Could you check a few things on this model? Use its own coordinates, in mm. Face numbers are marked on the shaded views. Coordinates: 2 decimals unless noted, no trailing zeros. Order: outer loops, then holes, each group sorted by start corner. A loop starts at its lowest first (then second) coordinate and runs counter-clockwise, first axis right, second up. Notation, with made-up numbers: (24, 50.25) - (54, 50.25) arc R25 ccw to (54, 69.25) - close; hole circle Ø2 at (47.5, 21). An arc over 180 degrees is marked (long way). One line per item, written item: value.
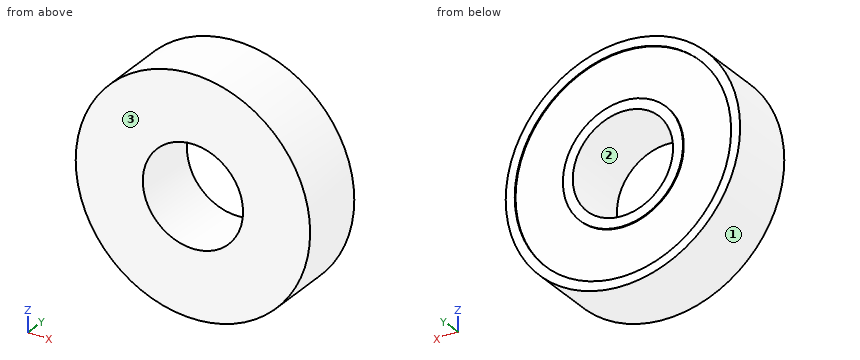
from build123d import *

# Parameters (mm, degrees)
CROQUIS1_R              = 13.975
SALIENTE_EXTRUIR1_DEPTH = 8
CROQUIS2_R              = 5.98
CORTAR_EXTRUIR1_DEPTH   = 8
CROQUIS3_R              = 7.163309877
CROQUIS3_R_2            = 5.98
SALIENTE_EXTRUIR3_DEPTH = 0.15
CROQUIS4_R              = 13.975
CROQUIS4_R_2            = 12.899809837
SALIENTE_EXTRUIR4_DEPTH = 8.15


with BuildPart() as part:
    # Croquis1 → Saliente-Extruir1 (new body)
    with BuildSketch(Plane(origin=(0, 0, 0), x_dir=(1, 0, 0), z_dir=(0, 1, 0))):
        Circle(CROQUIS1_R)
    extrude(amount=SALIENTE_EXTRUIR1_DEPTH)

    # Croquis2 → Cortar-Extruir1 (cut)
    with BuildSketch(Plane(origin=(0, 8, 0), x_dir=(1, 0, 0), z_dir=(0, 1, 0))):
        Circle(CROQUIS2_R)
    extrude(amount=-CORTAR_EXTRUIR1_DEPTH, mode=Mode.SUBTRACT)

    # Croquis3 → Saliente-Extruir3 (add)
    with BuildSketch(Plane(origin=(0, 8, 0), x_dir=(1, 0, 0), z_dir=(0, 1, 0))):
        Circle(CROQUIS3_R)
        Circle(CROQUIS3_R_2, mode=Mode.SUBTRACT)
    extrude(amount=SALIENTE_EXTRUIR3_DEPTH)

    # Croquis4 → Saliente-Extruir4 (add)
    with BuildSketch(Plane(origin=(0, 0, 0), x_dir=(1, 0, 0), z_dir=(0, 1, 0))):
        Circle(CROQUIS4_R)
        Circle(CROQUIS4_R_2, mode=Mode.SUBTRACT)
    extrude(amount=SALIENTE_EXTRUIR4_DEPTH)


solid = part.part
Item 1: I want a section at D-D on z = 8. Please give me the cut outline in (x, y).
Conclusion:
outline: (-11.46, 0) - (11.46, 0) - (11.46, 8.15) - (10.12, 8.15) - (10.12, 8) - (-10.12, 8) - (-10.12, 8.15) - (-11.46, 8.15) - close
Item 2: I want a section at C-C on y = 7. Please give me the cut outline in (x, z) (3 decimals).
Conclusion:
outline: circle Ø27.95 at (0, 0); hole circle Ø11.96 at (0, 0)
Item 3: I'm going to push flat-ended pins straight in: pin 1 Ø9.5 at (x, z) = (0, 0) entering from -Y; pin 2 Ø4 at (y, z) = (5, 6.5) entering from -X; pin 3 Ø3 at (y, z) = (6.5, 10.5) entering from -X; pin 4 Ø2 at (x, y) = (-10, 4) entering from -Z. Where does each tip first touch, or does it pass through?
Conclusion:
pin 1: through
pin 2: x = -13.23
pin 3: x = -10.69
pin 4: z = -10.69
Item 4: If I drill on probe 1 along X at (y, z) = (8.1, 0) (3 decimals); probe 2 along X at (y, z) = (2.5, 0) (3 decimals); probe 3 along X at (y, z) = (2.5, -2.25), over which ranges is the centre line in solid material (lowest first)?
Conclusion:
probe 1: -13.975 to -12.9, -7.163 to -5.98, 5.98 to 7.163, 12.9 to 13.975
probe 2: -13.975 to -5.98, 5.98 to 13.975
probe 3: -13.79 to -5.54, 5.54 to 13.79
Item 5: Thinking about a two-plate mould opening in Z: for the marked faces 1, 2 and 3, which applies, pulls with the +Z half, pulls with the -Z half, needs draft (parallel to the pull), parting line crosses it, or undercut?
Conclusion:
face 1: parting line crosses it
face 2: undercut
face 3: needs draft
Item 6: I want a section at B-B on x = 0. Please give me the cut outline in (y, z) (3 decimals).
Conclusion:
outline: (0, -13.975) - (8.15, -13.975) - (8.15, -12.9) - (8, -12.9) - (8, -7.163) - (8.15, -7.163) - (8.15, -5.98) - (0, -5.98) - close; (0, 5.98) - (8.15, 5.98) - (8.15, 7.163) - (8, 7.163) - (8, 12.9) - (8.15, 12.9) - (8.15, 13.975) - (0, 13.975) - close
Item 7: I want a section at A-A on z = 0. Please give me the cut outline in (x, y) (3 decimals), then the cut area to 3 significant figures.
Conclusion:
outline: (-13.975, 0) - (-5.98, 0) - (-5.98, 8.15) - (-7.163, 8.15) - (-7.163, 8) - (-12.9, 8) - (-12.9, 8.15) - (-13.975, 8.15) - close; (5.98, 0) - (13.975, 0) - (13.975, 8.15) - (12.9, 8.15) - (12.9, 8) - (7.163, 8) - (7.163, 8.15) - (5.98, 8.15) - close
area: 129 mm²
